Input: part model. Units: mm. Frame: model coordinates. Face numbers are marked on the shaded views. Give positions to 0.01 mm unless a question says otherwise; leave off trailing zeros. Loops run counter-clockwise (first coordinate to the right, second up) from the corner with the lowest first, then second, coordinate; pieces in that order, holes last. Notation, with made-up numbers: M 50,3.25 L 71,3.25 A19 cw 71,33.25 Z; hole C -7.5,-38 d11. An arc over 180 degrees is marked long. Answer as a JSON object with one key per item and string values. Group by question number.
1) Ray query, L1, parallel to X at y = -10.5, z = 0; L2, parallel to Z at x = 22.5, y = -17.75; L3, parallel to X at y = -10.25, z = -43. Return the intervals inside material, ascending.
2) First-contact query: P1, Ø5, axis at x = 13, z = -11, coming from the +Y side; P2, Ø12.5, axis at y = -6.5, z = 47, coming from the -X side; P3, Ø1.9, axis at y = -13.5, z = 54.5, coming from the -X side; P4, Ø7, axis at y = -18.5, z = 27, coming from the +X side. Flat tips, straight axial feed; report the tip coordinate or a pass-through.
3) Section query C-C on x = -55. Return loops of the section in (y, z).
4) Draft query along Z for the marked faces 1, 2 and 3. Return one class per face: +Z half, -Z half, draft (parallel to the pull), parting line (faces both ways), or undercut.
5) Section query D-D on z = -15.5. Count the separate pieces of the cut face and the enclosed holes in it, plus the area to 3 significant figures.
6) Section query B-B on z = 75. Return loops of the section in (x, y).
7) Section query A-A on x = 12. Return loops of the section in (y, z).
from build123d import *

# Parameters (mm, degrees)
F1_DEPTH = 25


with BuildPart() as f1:
    # F0 (on Front) → F1 (new body)
    with BuildSketch(Plane.XZ):
        with BuildLine():
            ThreePointArc((-29.977737, 52.477247), (-61.508504, 65.006824), (-84.561244, 40.112031))
            Line((-84.561244, 40.112031), (-84.561244, -5.112031))
            ThreePointArc((-84.561244, -5.112031), (-75.261665, -22.123854), (-57.499819, -29.895667))
            ThreePointArc((-57.499819, -29.895667), (-33.669065, -59.35886), (0.004668, -41.978865))
            ThreePointArc((0.004668, -41.978865), (33.690375, -59.336998), (57.501353, -29.857023))
            ThreePointArc((57.501353, -29.857023), (77.031456, -20.271453), (84.929231, 3.5e-05))
            Line((84.929231, 3.5e-05), (85.082121, 38.974539))
            ThreePointArc((85.082121, 38.974539), (62.093064, 64.528697), (29.975545, 52.282199))
            Line((29.975545, 52.282199), (29.97973, 58.897384))
            ThreePointArc((29.97973, 58.897384), (-0.026483, 89.999988), (-29.977737, 58.844456))
            Line((-29.977737, 58.844456), (-29.977737, 52.477247))
        make_face()
        with BuildLine():
            ThreePointArc((-52.499782, -29.895634), (-37.531172, -24.389343), (-27.5, -11.989579))
            ThreePointArc((-27.5, -11.989579), (-17.468828, -24.389343), (-2.500218, -29.895634))
            ThreePointArc((-2.500218, -29.895634), (-27.5, -55), (-52.499782, -29.895634))
        make_face(mode=Mode.SUBTRACT)
        with BuildLine():
            ThreePointArc((-57.06582, -24.914502), (-71.893116, 18.428854), (-30.000218, -0.104366))
            ThreePointArc((-30.000218, -0.104366), (-47.771739, -7.885376), (-57.06582, -24.914502))
        make_face(mode=Mode.SUBTRACT)
        with BuildLine():
            ThreePointArc((-51.956196, -24.814013), (-44.393116, -11.571146), (-30.543804, -5.185987))
            ThreePointArc((-30.543804, -5.185987), (-38.106884, -18.428854), (-51.956196, -24.814013))
        make_face(mode=Mode.SUBTRACT)
        with BuildLine():
            ThreePointArc((-3.043804, -24.814013), (-16.893116, -18.428854), (-24.456196, -5.185987))
            ThreePointArc((-24.456196, -5.185987), (-10.606884, -11.571146), (-3.043804, -24.814013))
        make_face(mode=Mode.SUBTRACT)
        with BuildLine():
            ThreePointArc((-24.999782, -0.104366), (-0.008793, 24.999998), (24.999849, -0.08678))
            ThreePointArc((24.999849, -0.08678), (10.027405, -5.596797), (-0.003054, -18.003419))
            ThreePointArc((-0.003054, -18.003419), (-10.034277, -5.608433), (-24.999782, -0.104366))
        make_face(mode=Mode.SUBTRACT)
        with BuildLine():
            ThreePointArc((2.501765, -29.895504), (17.471102, -24.387714), (27.501614, -11.985875))
            ThreePointArc((27.501614, -11.985875), (37.534897, -24.373797), (52.501331, -29.863173))
            ThreePointArc((52.501331, -29.863173), (27.51778, -54.982279), (2.501765, -29.895504))
        make_face(mode=Mode.SUBTRACT)
        with BuildLine():
            ThreePointArc((3.041611, -24.814282), (10.602538, -11.558896), (24.460003, -5.168002))
            ThreePointArc((24.460003, -5.168002), (16.899076, -18.423388), (3.041611, -24.814282))
        make_face(mode=Mode.SUBTRACT)
        with BuildLine():
            ThreePointArc((51.954881, -24.782502), (38.102344, -18.409101), (30.540719, -5.167695))
            ThreePointArc((30.540719, -5.167695), (44.387786, -11.547068), (51.954881, -24.782502))
        make_face(mode=Mode.SUBTRACT)
        with BuildLine():
            ThreePointArc((30.00015, -0.08651), (71.826887, 18.409146), (57.063881, -24.876173))
            ThreePointArc((57.063881, -24.876173), (47.76502, -7.860024), (30.00015, -0.08651))
        make_face(mode=Mode.SUBTRACT)
        with BuildLine():
            Line((-31.048497, 42.16418), (-31.048497, 18.064481))
            ThreePointArc((-31.048497, 18.064481), (-55.31332, 29.998364), (-79.323589, 17.560269))
            Line((-79.323589, 17.560269), (-79.323589, 40.776075))
            ThreePointArc((-79.323589, 40.776075), (-55.718555, 59.989671), (-31.048497, 42.16418))
        make_face(mode=Mode.SUBTRACT)
        with BuildLine():
            Line((24.859272, 57.35111), (24.859272, 16.79335))
            ThreePointArc((24.859272, 16.79335), (-0.120786, 29.999757), (-24.993691, 16.592631))
            Line((-24.993691, 16.592631), (-24.993691, 59.438392))
            ThreePointArc((-24.993691, 59.438392), (1.045803, 84.978116), (24.859272, 57.35111))
        make_face(mode=Mode.SUBTRACT)
        with BuildLine():
            ThreePointArc((29.965727, 34.764301), (29.964616, 35.000022), (29.965727, 35.235743))
            ThreePointArc((29.965727, 35.235743), (54.603474, 59.997414), (79.946261, 35.95782))
            ThreePointArc((79.946261, 35.95782), (79.964616, 35.000022), (79.946261, 34.042225))
            Line((79.946261, 34.042225), (79.946261, 16.546791))
            ThreePointArc((79.946261, 16.546791), (54.948991, 29.964634), (29.965727, 16.520729))
            Line((29.965727, 16.520729), (29.965727, 34.764301))
        make_face(mode=Mode.SUBTRACT)
    extrude(amount=F1_DEPTH)


solid = f1.part
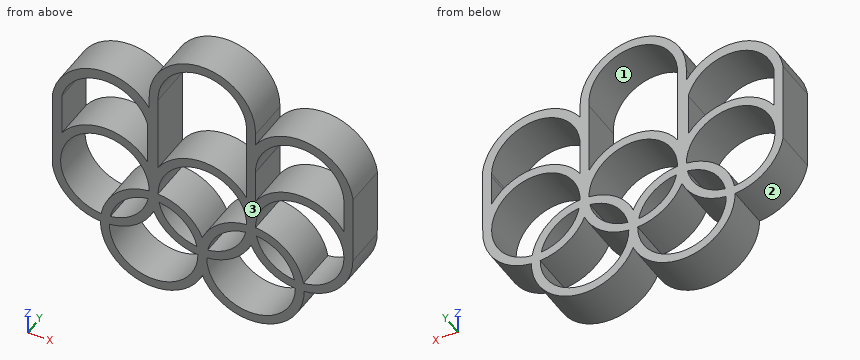
Output:
{
 "1": {"L1": "x = -84.56 to -80, -30 to -25, 25 to 30, 79.93 to 84.93", "L2": "z = -59.56 to -54.48, -19.84 to -10.9, -5.49 to -0.4, 10.9 to 19.84, 70.9 to 79.84", "L3": "x = -54.54 to -48.85, -6.15 to -0.46, 0.47 to 6.16, 48.84 to 54.53"},
 "2": {"P1": "stops at y = 0", "P2": "stops at x = -84.46", "P3": "stops at x = -79.03", "P4": "stops at x = 85.05"},
 "3": {"outline": "M -25,-41.99 L 0,-41.99 L 0,-18.01 L -25,-18.01 Z; M -25,25 L 0,25 L 0,30 L -25,30 Z; M -25,60 L 0,60 L 0,65.75 L -25,65.75 Z"},
 "4": {"face 1": "undercut", "face 2": "-Z half", "face 3": "draft"},
 "5": {"separate pieces": "10", "enclosed holes": "0", "area": "1,500 mm^2"},
 "6": {"outline": "M -25.98,-25 L -20,-25 L -20,0 L -25.98,0 Z; M 20,-25 L 25.98,-25 L 25.98,0 L 20,0 Z"},
 "7": {"outline": "M -25,-55.67 L 0,-55.67 L 0,-49.6 L -25,-49.6 Z; M -25,-27.5 L 0,-27.5 L 0,-21.93 L -25,-21.93 Z; M -25,-10.37 L 0,-10.37 L 0,-4.3 L -25,-4.3 Z; M -25,21.93 L 0,21.93 L 0,27.5 L -25,27.5 Z; M -25,81.93 L 0,81.93 L 0,87.5 L -25,87.5 Z"}
}
